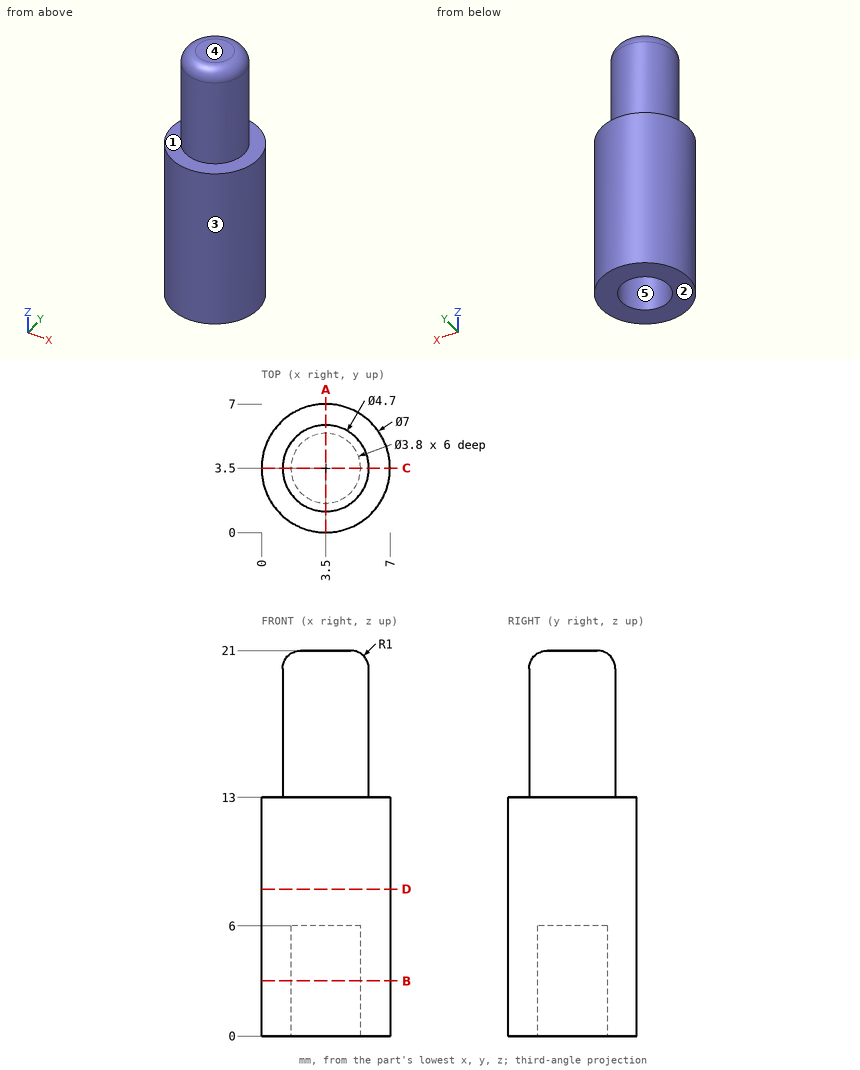
Design review of the part shown in the three views and the two pictorial views. Dimensions are in mm from the part's minimum x, y and z. A direction names the side the tool comes from. Give positions to 0.01 mm unless a question says otherwise; leave off trailing zeros. Write each loop counter-clockwise with the first axis right and the second up, starting at its lowest first coordinate (ties: lowest second). Pieces come first, ordered by that corner, then holes. Notation, with made-up numbers: M 20.25,22 L 52.25,22 A24 ccw 52.25,52 Z; hole C 70.25,-36 d5. An arc over 180 degrees is marked long. One line per question, with ' | ' between items. Start each with the question number.
Item 1: We need section B-B on z = 3. Write out the cut boundary in (x, y), plus the area to 3 significant figures.
Item 2: Wall thickness on line 1 (Y direction, x = 3.5, z = 1.65); line 2 (Z direction, x = 3, y = 3.5); line 3 (Z direction, x = 6, y = 3): over which ranges is each line inside the solid? List them lowest first. Write a range as from..to.
Item 3: Draft analysis for pull direction X (two halves, no side actions). For the marked faces 3, 4 and 5, state which applies: released by +X, released by -X, zero draft, split by the parting line, or undercut.
Item 4: We need section D-D on z = 8. Write out the cut boundary in (x, y), plus the area to 3 significant figures.
Item 5: For the marked faces 1 and 2, list the 3-axis set-ups (+Z, -Z, +X, -X, +Y, -Y) from which the entire face can be reached by the end or side of a thin tool; tool diameter is ignored.
Item 6: For pin 1 (1 mm diameter, centred on x = 4.5, z = 3.5, fed in from -Y); pin 2 (4 mm diameter, centred on y = 3, z = 15.5, fed in from +X), all flat-tipped, find the tip position at first contact; note any pin that passes through.
Item 7: We need section A-A on x = 3.5. Write out the cut boundary in (y, z), plus the area to 3 significant figures.
Results found:
1) outline: C 3.5,3.5 d7; hole C 3.5,3.5 d3.8 | area: 27.1 mm2
2) line 1: y = 0..1.6, 5.4..7 | line 2: z = 6..21 | line 3: z = 0..13
3) face 3: split by the parting line | face 4: zero draft | face 5: undercut
4) outline: C 3.5,3.5 d7 | area: 38.5 mm2
5) face 1: +Z | face 2: -Z, +X, -X, +Y, -Y
6) pin 1: stops at y = 0.04 | pin 2: stops at x = 5.85
7) outline: M 0,0 L 1.6,0 L 1.6,6 L 5.4,6 L 5.4,0 L 7,0 L 7,13 L 5.85,13 L 5.85,20 A1 ccw 4.85,21 L 2.15,21 A1 ccw 1.15,20 L 1.15,13 L 0,13 Z | area: 105 mm2
